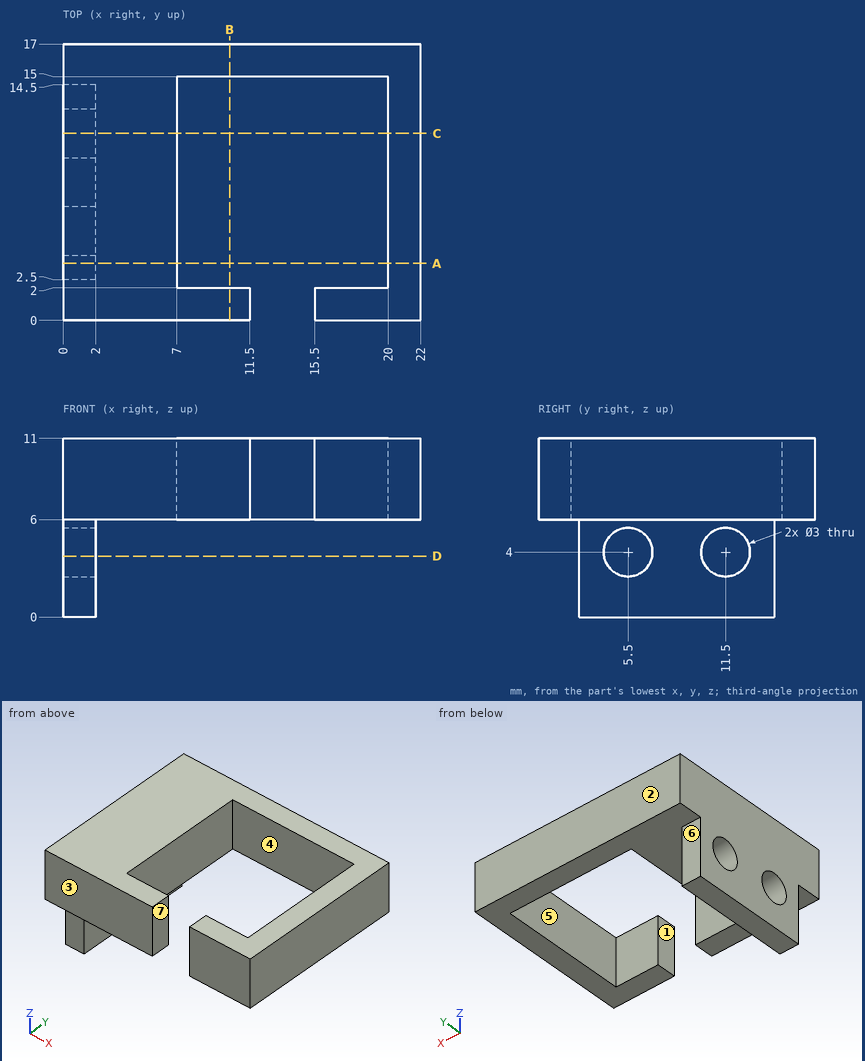
Could you check a few things on this drawing? It's one solid part, dimensions in mm from its lowest x, y, z. A direction names the side the tool comes from. Give positions to 0.01 mm unless a question says otherwise; leave off trailing zeros. Write each loop counter-clockwise with the first axis right and the second up, starting at its lowest first coordinate (ties: lowest second). Pieces come first, ordered by that corner, then holes. Notation, with made-up numbers: M 67,-36 L 122,-36 A24 ccw 122,-18 Z; hole C 64,39 d7. An arc over 180 degrees is marked long. Put each result on its own line as item: value. Start each with the question number.
Item 1: If we section it at D-D, the plane z = 3.75: Write out the boundary of the cut face in (x, y).
Item 2: I need wall thicknesses on L1, parallel to Y at x = 1.55, z = 4; L2, parallel to Z at x = 0.55, y = 5.5; L3, parallel to X at y = 8.25, z = 6.5. Which ranges of each line are inside material? Lowest first, please. Write a range as from..to.
Item 3: If we section it at B-B, the plane x = 10.25: Write out the boundary of the cut face in (y, z).
Item 4: If we section it at C-C, the plane y = 11.5: Write out the boundary of the cut face in (x, z).
Item 5: If we section it at A-A, the plane y = 3.5: Write out the boundary of the cut face in (x, z), then the cut area to 3 significant figures.
Item 6: Thinking about a two-plate mould opening in Y: for the marked faces 1, 2, 3 and 4, which applies, +Y half, -Y half, draft (parallel to the pull), parting line (faces both ways), or undercut?
Item 7: On a 3-axis mill with a long thin cutter (end or side, diameter ignored), from which of +Z, -Z, +X, -X, +Y, -Y can I reach the whole of each face in a straight line? I mean the marked faces 5, 6 and 7. Say none if no direction works.
Item 8: Will these pins go through, and if not, where does the flat tip stop? pin 1 (4 mm diameter, centred on x = 4.5, z = 1.5, fed in from -Y); pin 2 (6.5 mm diameter, centred on y = 7, z = 1.5, fed in from +X); pin 3 (1.6 mm diameter, centred on x = 1.5, z = 4, fed in from -Y); pin 4 (1.6 mm diameter, centred on x = 1.5, z = 2.5, fed in from +Y).
Values:
1. outline: M 0,2.5 L 2,2.5 L 2,4.02 L 0,4.02 Z; M 0,6.98 L 2,6.98 L 2,10.02 L 0,10.02 Z; M 0,12.98 L 2,12.98 L 2,14.5 L 0,14.5 Z
2. L1: 2.5..4, 7..10, 13..14.5
2. L2: 0..2.5, 5.5..11
2. L3: 0..7, 20..22
3. outline: M 0,6 L 2,6 L 2,11 L 0,11 Z; M 15,6 L 17,6 L 17,11 L 15,11 Z
4. outline: M 0,0 L 2,0 L 2,2.5 L 0,2.5 Z; M 0,5.5 L 2,5.5 L 2,6 L 7,6 L 7,11 L 0,11 Z; M 20,6 L 22,6 L 22,11 L 20,11 Z
5. outline: M 0,0 L 2,0 L 2,6 L 7,6 L 7,11 L 0,11 Z; M 20,6 L 22,6 L 22,11 L 20,11 Z
5. area: 57.0 mm²
6. face 1: draft
6. face 2: +Y half
6. face 3: -Y half
6. face 4: undercut
7. face 5: +Z, -Z
7. face 6: -Z, +X, -X, +Y
7. face 7: +Z, -Z, -Y
8. pin 1: through
8. pin 2: x = 2
8. pin 3: y = 2.5
8. pin 4: y = 14.5
